For this review, take the finished solid that the model builds, in its own axes (mm). A direction names the side the tool comes from. Coordinates: 2 decimals unless noted, no trailing zeros. Loops run counter-clockwise (first coordinate to the right, second up) from the corner with the lowest first, then second, coordinate; pieces in that order, holes last. Notation, with made-up numbers: (-20.75, 12) - (-3.75, 12) arc R13 cw to (-3.75, 34) - close; hole circle Ø7 at (74, 34). An arc over 180 degrees is marked (long way). Use one line per item in the form item = value. Start each with the question number.
1. Add section A-A on z = -3.5. Give the boundary of the cut face in (x, y), and give its area (3 significant figures).
2. For pin 1 Ø2 at (x, z) = (-0.5, -1) entering from +Y; pin 2 Ø1 at (y, z) = (14, -2) entering from -X, all flat-tipped, find the tip position at first contact; note any pin that passes through.
3. Machinability: for faces 5 (the face through (0.798, 13.955, -1.855)), 6 (the face through (5, 6, -2)), which of the approach directions +Z, -Z, +X, -X, +Y, -Y give a long, thin tool a straight path to every point of the face, cutting with its end or side? Answer none if there is none.
4. Draft analysis for pull direction Y (two halves, no side actions). For faces 1 (the face through (1.114, 15.983, -1.591)), 2 (the face through (0, 6, -2)), 3 (the face through (2.521, 17.623, -0.259)), 4 (the face through (-2, 0, -1)), state which applies: +Y half, -Y half, draft (parallel to the pull), parting line (faces both ways), or undercut.
5. Add section B-B on y = -1. Give the boundary of the cut face in (x, z) (3 decimals).
6. To check wall thickness, follow probe 1 along X at (y, z) = (8.5, -3.75); probe 2 along Z at (x, y) = (1.5, 9.75); probe 3 along Z at (x, y) = (1, 0.5). State the ranges of each line that lie inside material, in increasing order.
7. Add section D-D on y = 9.75. Give the boundary of the cut face in (x, z), and give its area (3 significant figures).
8. Add section C-C on x = -2.25. Give the boundary of the cut face in (y, z), and give its area (3 significant figures).
```python
from build123d import *

# Parameters (mm, degrees)
F1_DEPTH = 5
F2_R     = 1.5
F3_DEPTH = 4
F4_R     = 1.5
F5_DEPTH = 4


with BuildPart() as f1:
    # F0 (on Right) → F1 (new body)
    with BuildSketch(Plane.YZ):
        Polygon((9.999834287, 0.0575693728), (0, 0), (0, -5), (9.999834287, -5.0575693728), (14.9176799717, -4.1549100676), (12.9655016395, 0.510136665), align=None)
        with BuildLine():
            Line((0, -5), (0, 0))
            ThreePointArc((0, 0), (-2.4856488472, -2.5), (0, -5))
        make_face()
    extrude(amount=F1_DEPTH)

    # F2 (on face) → F3 (join)
    with BuildSketch(Plane(origin=(0, 0, 0), x_dir=(0, -1, 0), z_dir=(-1, 0, 0))):
        with Locations((-0.0143925817, -2.5)):
            Circle(F2_R)
    extrude(amount=F3_DEPTH)

    # F4 (on face) → F5 (join)
    with BuildSketch(Plane(origin=(0, 11.2150399751, 4.6931487054), x_dir=(-1, 0, 0), z_dir=(0, 0.9224854916, 0.3860317574))):
        with Locations((-2.5, -7.0630220916)):
            Circle(F4_R)
    extrude(amount=F5_DEPTH)


solid = f1.part
```
Conclusion:
q1.outline = (-4, -1.1) - (0, -1.1) - (0, -2.28) - (5, -2.28) - (5, 14.64) - (0, 14.64) - (0, 1.13) - (-4, 1.13) - close
q1.area = 93.5 mm^2
q2.pin_1 = 13.96
q2.pin_2 = 0
q3.face_5 = none
q3.face_6 = +Z, -Z, +X, +Y, -Y
q4.face_1 = undercut
q4.face_2 = draft
q4.face_3 = +Y half
q4.face_4 = parting line
q5.outline = (-4, -3.605) - (0, -3.605) - (0, -4.785) - (5, -4.785) - (5, -0.215) - (0, -0.215) - (0, -1.395) - (-4, -1.395) - close
q6.probe_1 = 0 to 5
q6.probe_2 = -5.06 to 0.06
q6.probe_3 = -5 to 0
q7.outline = (0, -5.06) - (5, -5.06) - (5, 0.06) - (0, 0.06) - close
q7.area = 25.6 mm^2
q8.outline = circle Ø3 at (0.01, -2.5)
q8.area = 7.07 mm^2
